from build123d import *

# Parameters (mm, degrees)
SKETCH_1_W          = 33
SKETCH_1_H          = 28
SKETCH_1_W_2        = 17
SKETCH_1_H_2        = 8
EXTRUDE_1_DEPTH     = 5
SKETCH_2_W          = 8
SKETCH_2_H          = 18
EXTRUDE_2_DEPTH     = 15
SKETCH_3_R          = 4.2
CUT_EXTRUDE_1_DEPTH = 37
FILLET_1_R          = 9
FILLET_2_R          = 1
SKETCH_4_R          = 2.25
CUT_EXTRUDE_2_DEPTH = 37


with BuildPart() as part:
    # 草图1 → 凸台-拉伸1 (new body)
    with BuildSketch(Plane(origin=(0, 0, 0), x_dir=(1, 0, 0), z_dir=(0, 1, 0))):
        with Locations((0, -5)):
            Rectangle(SKETCH_1_W, SKETCH_1_H)
        Rectangle(SKETCH_1_W_2, SKETCH_1_H_2, mode=Mode.SUBTRACT)
    extrude(amount=EXTRUDE_1_DEPTH)

    # 草图2 → 凸台-拉伸2 (add)
    with BuildSketch(Plane.XZ):
        with Locations((-12.5, 0)):
            Rectangle(SKETCH_2_W, SKETCH_2_H)
        with Locations((12.5, 0)):
            Rectangle(SKETCH_2_W, SKETCH_2_H)
    extrude(amount=EXTRUDE_2_DEPTH)

    # 草图3 → 切除-拉伸1 (cut)
    with BuildSketch(Plane.ZY.offset(16.5)):
        with Locations((0, -8)):
            Circle(SKETCH_3_R)
    extrude(amount=-CUT_EXTRUDE_1_DEPTH, mode=Mode.SUBTRACT)

    # 圆角1
    fillet_1_edges = [part.edges().sort_by_distance(p)[0] for p in [
        (12.5, -15, -9),
        (12.5, -15, 9),
        (-12.5, -15, 9),
        (-12.5, -15, -9),
    ]]
    fillet(fillet_1_edges, radius=FILLET_1_R - 0.0001)  # a hair under: the kernel refuses the full size

    # 圆角2
    fillet_2_edges = [part.edges().sort_by_distance(p)[0] for p in [
        (-8.5, 0, 6.5),
        (-8.5, 0, -6.5),
        (-12.5, 0, 9),
        (12.5, 0, 9),
        (8.5, 0, 6.5),
        (8.5, 0, -6.5),
    ]]
    fillet(fillet_2_edges, radius=FILLET_2_R)

    # 草图4 → 切除-拉伸2 (cut)
    with BuildSketch(Plane.XZ):
        with Locations(Location((-12.5, 14.5, 0), (0, 0, 270))):
            Circle(SKETCH_4_R)
        with Locations(Location((12.5, 14.5, 0), (0, 0, 270))):
            Circle(SKETCH_4_R)
    extrude(amount=-CUT_EXTRUDE_2_DEPTH, mode=Mode.SUBTRACT)


solid = part.part
Design review of the part built by this model. Coordinates are the model's own, in mm. A direction names the side the tool comes from. Coordinates: 2 decimals unless noted, no trailing zeros. Loops run counter-clockwise (first coordinate to the right, second up) from the corner with the lowest first, then second, coordinate; pieces in that order, holes last. Notation, with made-up numbers: (23.25, 47) -> (49.25, 47) arc R21 ccw to (49.25, 56) -> close; hole circle Ø2 at (-1.5, 10). An arc over 180 degrees is marked (long way). Use a Markdown table: item, result. Add a question column.
Item 1: We need section B-B, the plane z = 14.5. Write out the cut boundary in (x, y), and give its area (3 significant figures).
Item 2: Wall thickness on L1, parallel to X at y = 3.75, z = 14.5; L2, parallel to X at y = -11.25, z = 6; L3, parallel to Y at x = 10.5, z = 0: over which ranges is each line inside the solid? List them lowest first. Write a range as from..to.
Item 3: We need section A-A, the plane x = 6. Write out the cut boundary in (y, z), and give its area (3 significant figures).
Item 4: The part is to be moulded in two halves that separate along Z. For faces 6 (the cylindrical face through (-12.56, -12.1, -0.91)), 7 (the flat face through (0, 1, -9)), 8 (the flat face through (0, 2, 19)), 9 (the flat face through (0, 5, 5)), say which applies: +Z half, -Z half, draft (parallel to the pull), parting line (faces both ways), or undercut.
Item 5: Clearance check with flat-ended pins moving along their axes: P1, Ø3.5, axis at x = -12.5, z = 14.5, coming from the -Y side; P2, Ø4, axis at x = -2.5, z = -7.5, coming from the -Y side; P3, Ø1.5, axis at x = -13, y = -4, coming from the +Z side; P4, Ø16.5, axis at x = 8, z = 11.5, coming from the -Y side. State where each tip first meets the part, or that it passes through.
Item 6: We need section C-C, the plane x = -12. Count the separate pieces of the cut face and the enclosed holes in it, and give its area (3 significant figures).
Item 7: We need section D-D, the plane y = 1.25. Write out the cut boundary in (x, z).
Item 8: Machinability: for faces 1 (the flat face through (8.5, -3, 0)), 2 (the flat face through (0, 0, 13)), 3 (the cylindrical face through (8.199, -0.285, -6.465)), 4 (the flat face through (0, 3, 4)), 5 (the cylindrical face through (12.556, -12.294, -6.434)), which of the approach directions +Z, -Z, +X, -X, +Y, -Y give a long, thin tool a straight path to every point of the face, cutting with its end or side? Answer none if there is none.
Numbers:
| question | item | result |
|---|---|---|
| 1 | outline | (-16.5, 0) -> (-14.75, 0) -> (-14.75, 5) -> (-16.5, 5) -> close; (-10.25, 0) -> (10.25, 0) -> (10.25, 5) -> (-10.25, 5) -> close; (14.75, 0) -> (16.5, 0) -> (16.5, 5) -> (14.75, 5) -> close |
| 1 | area | 120 mm^2 |
| 2 | L1 | x = -16.5..-14.75, -10.25..10.25, 14.75..16.5 |
| 2 | L2 | x = -16.5..-8.5, 8.5..16.5 |
| 2 | L3 | y = -15..-12.2, -3.8..5 |
| 3 | outline | (0, -9) -> (5, -9) -> (5, -4) -> (0, -4) -> close; (0, 4) -> (5, 4) -> (5, 19) -> (0, 19) -> close |
| 3 | area | 100 mm^2 |
| 4 | face 6 | undercut |
| 4 | face 7 | -Z half |
| 4 | face 8 | +Z half |
| 4 | face 9 | draft |
| 5 | P1 | passes through |
| 5 | P2 | stops at y = 0 |
| 5 | P3 | stops at z = 9 |
| 5 | P4 | stops at y = -14.39 |
| 6 | separate pieces | 2 |
| 6 | enclosed holes | 1 |
| 6 | area | 298 mm^2 |
| 7 | outline | (-16.5, -9) -> (16.5, -9) -> (16.5, 19) -> (-16.5, 19) -> close; hole circle Ø4.5 at (-12.5, 14.5); hole (-8.5, -4) -> (8.5, -4) -> (8.5, 4) -> (-8.5, 4) -> close; hole circle Ø4.5 at (12.5, 14.5) |
| 8 | face 1 | -Y |
| 8 | face 2 | +Z, -Y |
| 8 | face 3 | +Z, -Z, -Y |
| 8 | face 4 | +Y, -Y |
| 8 | face 5 | -Z, +X, -X, -Y |
